Here's how the part is built. I have some questions about the finished solid (model axes, mm). Face numbers are marked on the shaded views. A direction names the side the tool comes from. Round coordinates to 2 decimals unless told otherwise and drop trailing zeros. Order: outer loops, then holes, each group sorted by start corner. A loop starts at its lowest first (then second) coordinate and runs counter-clockwise, first axis right, second up. Notation, with made-up numbers: (11, 81.25) -> (33, 81.25) arc R20 ccw to (33, 110.25) -> close; hole circle Ø3 at (77.5, -14.5). An arc over 180 degrees is marked (long way). One line per item, written item: value.
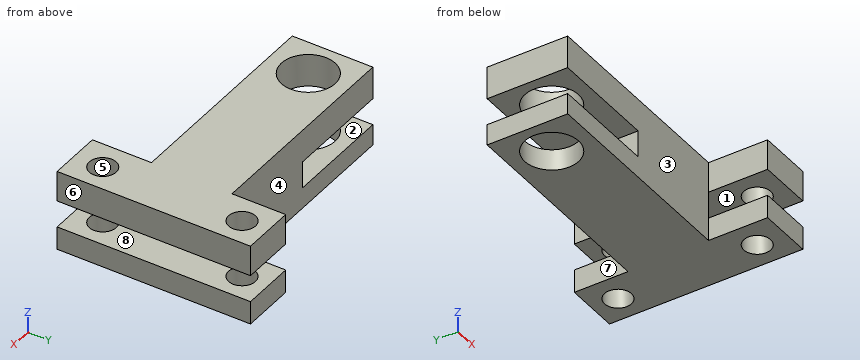
```python
from build123d import *

# Parameters (mm, degrees)
SKETCH1_W           = 50
SKETCH1_H           = 15
BOSS_EXTRUDE1_DEPTH = 15
SKETCH3_W           = 20
SKETCH3_H           = 5
CUT_EXTRUDE1_DEPTH  = 30
SKETCH5_R           = 5
CUT_EXTRUDE2_DEPTH  = 30
SKETCH7_W           = 10
SKETCH7_H           = 15
BOSS_EXTRUDE2_DEPTH = 10
SKETCH11_W          = 10
SKETCH11_H          = 15
BOSS_EXTRUDE5_DEPTH = 11
SKETCH12_R          = 2.5
CUT_EXTRUDE3_DEPTH  = 25
SKETCH13_W          = 5
SKETCH13_H          = 36
CUT_EXTRUDE4_DEPTH  = 10


with BuildPart() as part:
    # Sketch1 → Boss-Extrude1 (new body)
    with BuildSketch(Plane.XY):
        Rectangle(SKETCH1_W, SKETCH1_H)
    extrude(amount=BOSS_EXTRUDE1_DEPTH)

    # Sketch3 → Cut-Extrude1 (cut)
    with BuildSketch(Plane(origin=(0, 7.5, 0), x_dir=(1, 0, 0), z_dir=(0, 1, 0))):
        with Locations((-15, -6.411378574)):
            Rectangle(SKETCH3_W, SKETCH3_H)
    extrude(amount=-CUT_EXTRUDE1_DEPTH, mode=Mode.SUBTRACT)

    # Sketch5 → Cut-Extrude2 (cut)
    with BuildSketch(Plane.XY.offset(15)):
        with Locations((-18.108253402, 0)):
            Circle(SKETCH5_R)
    extrude(amount=-CUT_EXTRUDE2_DEPTH, mode=Mode.SUBTRACT)

    # Sketch7 → Boss-Extrude2 (add)
    with BuildSketch(Plane(origin=(0, 7.5, 0), x_dir=(1, 0, 0), z_dir=(0, 1, 0))):
        with Locations((20, -7.5)):
            Rectangle(SKETCH7_W, SKETCH7_H)
    extrude(amount=BOSS_EXTRUDE2_DEPTH)

    # Sketch11 → Boss-Extrude5 (add)
    with BuildSketch(Plane.XZ.offset(7.5)):
        with Locations((20, 7.5)):
            Rectangle(SKETCH11_W, SKETCH11_H)
    extrude(amount=BOSS_EXTRUDE5_DEPTH)

    # Sketch12 → Cut-Extrude3 (cut)
    with BuildSketch(Plane.XY.offset(15)):
        with Locations((20.132117018, 12.735002854)):
            Circle(SKETCH12_R)
        with Locations((20.132117018, -13.202407166)):
            Circle(SKETCH12_R)
    extrude(amount=-CUT_EXTRUDE3_DEPTH, mode=Mode.SUBTRACT)

    # Sketch13 → Cut-Extrude4 (cut)
    with BuildSketch(Plane(origin=(25, 0, 0), x_dir=(0, 0, -1), z_dir=(1, 0, 0))):
        with Locations((-6.81082534, -0.5)):
            Rectangle(SKETCH13_W, SKETCH13_H)
    extrude(amount=-CUT_EXTRUDE4_DEPTH, mode=Mode.SUBTRACT)


solid = part.part
```
Q1. For P1, Ø3, axis at y = -14.5, z = 12.5, coming from the -X side; P2, Ø7.5, axis at x = -6.5, z = 7, coming from the -Y side; P3, Ø1, axis at x = -17, z = 10, coming from the +Y side, each with a flat end and sliding along its axis, tell me the tip position at first contact or that it passes through.
Answers:
P1: x = 15
P2: y = -7.5
P3: y = 7.5
Q2. Which directions (+Z, -Z, +X, -X, +Y, -Y) give clear straight access to the entire face, cutting with the end or side of a thin tool? Please do the marked faces 1, 2, 3 and 4.
Answers:
face 1: +X, +Y, -Y
face 2: -X, +Y, -Y
face 3: +Z, -Z, -X, -Y
face 4: +Z, -Z, -X, +Y
Q3. I want a section at A-A on y = 0. Write out the boundary of the cut face in (x, z), then the cut area to 3 significant figures.
Answers:
outline: (-25, 0) -> (-23.11, 0) -> (-23.11, 3.91) -> (-25, 3.91) -> close; (-25, 8.91) -> (-23.11, 8.91) -> (-23.11, 15) -> (-25, 15) -> close; (-13.11, 0) -> (25, 0) -> (25, 4.31) -> (15, 4.31) -> (15, 9.31) -> (25, 9.31) -> (25, 15) -> (-13.11, 15) -> (-13.11, 8.91) -> (-5, 8.91) -> (-5, 3.91) -> (-13.11, 3.91) -> close
area: 500 mm2
Q4. I want a section at C-C on y = 6. Write out the boundary of the cut face in (x, z), then the cut area to 3 significant figures.
Answers:
outline: (-25, 0) -> (25, 0) -> (25, 4.31) -> (15, 4.31) -> (15, 9.31) -> (25, 9.31) -> (25, 15) -> (-25, 15) -> (-25, 8.91) -> (-5, 8.91) -> (-5, 3.91) -> (-25, 3.91) -> close
area: 600 mm2
Q5. I want a section at B-B on x = -18. Write out the boundary of the cut face in (y, z), then the cut area to 3 significant figures.
Answers:
outline: (-7.5, 0) -> (-5, 0) -> (-5, 3.91) -> (-7.5, 3.91) -> close; (-7.5, 8.91) -> (-5, 8.91) -> (-5, 15) -> (-7.5, 15) -> close; (5, 0) -> (7.5, 0) -> (7.5, 3.91) -> (5, 3.91) -> close; (5, 8.91) -> (7.5, 8.91) -> (7.5, 15) -> (5, 15) -> close
area: 50.0 mm2
Q6. If we mould it in two halves opening along X, with no side actions, what happens to the marked faces 5, 6, 7 and 8? For each: pulls with the +X half, pulls with the -X half, needs draft (parallel to the pull), parting line crosses it, or undercut.
Answers:
face 5: undercut
face 6: pulls with the +X half
face 7: pulls with the -X half
face 8: needs draft
Q7. I want a section at D-D on z = 11. Write out the boundary of the cut face in (x, y) (3 decimals).
Answers:
outline: (-25, -7.5) -> (15, -7.5) -> (15, -18.5) -> (25, -18.5) -> (25, 17.5) -> (15, 17.5) -> (15, 7.5) -> (-25, 7.5) -> close; hole circle Ø10 at (-18.108, 0); hole circle Ø5 at (20.132, -13.202); hole circle Ø5 at (20.132, 12.735)
Q8. I need wall thicknesses on line 1 along Z through (x, y) = (-6, -0.5); line 2 along Z through (x, y) = (15.5, -2.5); line 3 along Y through (x, z) = (21, 13). Which ranges of each line are inside material? Lowest first, please.
Answers:
line 1: 0 to 3.91, 8.91 to 15
line 2: 0 to 4.31, 9.31 to 15
line 3: -18.5 to -15.55, -10.86 to 10.39, 15.08 to 17.5
